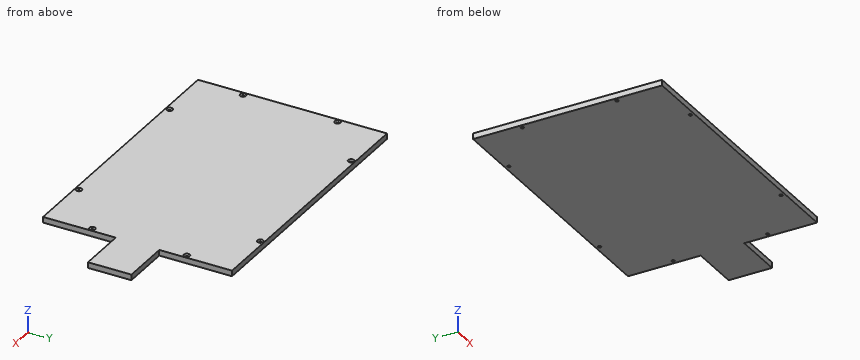
Autodesk Inventor part; units mm, degrees
ref_plane "YZ Plane" through (0, 0, 0) normal (1, 0, 0) x (0, 1, 0)
ref_plane "XZ Plane" through (0, 0, 0) normal (0, 1, 0) x (-1, 0, 0)
ref_plane "XY Plane" through (0, 0, 0) normal (0, 0, 1) x (1, 0, 0)
sketch "Skizze1" plane through (0, 0, 0) normal (0, 0, 1) x (1, 0, 0)
  line L0 (0, 120) -> (0, -20)
  line L1 (-68.3, 0) -> (409.8, 0)
  line L2 (0, 0) -> (217.779, 0)
  line L3 (289.5, 23) -> (289.5, 100)
  line L4 (289.5, 100) -> (0, 100)
  line L5 (0, 100) -> (0, 0)
  line L6 (217.779, 0) -> (341.5, 0)
  line L7 (341.5, 0) -> (341.5, 23)
  line L8 (341.5, 23) -> (289.5, 23)
  dimension "d0" = 52
  dimension "d1" = 289.5
  dimension "d2" = 100
  dimension "d3" = 23
extrude "Extrusion1" add sketch "Skizze1" along normal blind 6
mirror "Spiegeln1" about plane through (217.779, 0, 0) normal (0, -1, 0)
sketch "Skizze2" plane through (0, 0, 6) normal (0, 0, 1) x (1, 0, 0)
  line L0 (0, -100) -> (0, 100)
  line L1 (289.5, 100) -> (289.5, 23)
  line L2 (0, 100) -> (289.5, 100)
  point P0 (0, 0)
  point P1 (60, 96)
  point P2 (229.5, 96)
  point P3 (4, 50)
  point P4 (285.5, 50)
  dimension "d6" = 60
  dimension "d7" = 60
  dimension "d8" = 50
  dimension "d9" = 50
  dimension "d10" = 4
  dimension "d11" = 4
  dimension "d12" = 4
  dimension "d13" = 4
hole "Bohrung1" at (60, 96, 6) at (229.5, 96, 6) at (4, 50, 6) at (285.5, 50, 6) direction (0, 0, -1) diameter 3.2 end through all countersink diameter 6.2 countersink angle 90
mirror "Spiegeln2" about plane through (0, 0, 0) normal (0, 1, 0) of "Bohrung1"
properties part number "Deckel2" material "Polycarbonate, Clear"
Read the model definition and answer for the solid it produces. Units are mm, in the model's axes. Round coordinates to 2 decimals unless told otherwise and drop trailing zeros. Write each loop counter-clockwise with the first axis right and the second up, starting at its lowest first coordinate (ties: lowest second). Pieces come first, ordered by that corner, then holes.
Q1. Flat-ended cylindrical pins translate along their axes: P1, Ø3, axis at y = 59.5, z = 2.5, coming from the +X side; P2, Ø2, axis at x = 298, z = 5, coming from the +Y side; P3, Ø5, axis at x = 4, y = 50, coming from the +Z side. Find the tip coordinate at first contact, or state that the pin passes through.
Values:
P1: stops at x = 289.5
P2: stops at y = 23
P3: stops at z = 5.4
Q2. Find section B-B on y = -27.5. Determine the outline of the cut face in (x, z).
Values:
outline: (0, 0) - (289.5, 0) - (289.5, 6) - (0, 6) - close
Q3. Find section A-A on z = 2.25. State how many separate pieces and enclosed holes the cut face has, and give its area (3 significant figures).
Values:
separate pieces: 1
enclosed holes: 8
area: 60,200 mm2
Q4. Straight lines are drawn through the part: line 1 (X direction, y = 50, z = 1.1); line 2 (Y direction, x = 4, z = 3.3); line 3 (X direction, y = 96, z = 2.2). For each, find the intervals that lie inside material, in ascending order.
Values:
line 1: x = 0 to 2.4, 5.6 to 283.9, 287.1 to 289.5
line 2: y = -100 to -51.6, -48.4 to 48.4, 51.6 to 100
line 3: x = 0 to 58.4, 61.6 to 227.9, 231.1 to 289.5
